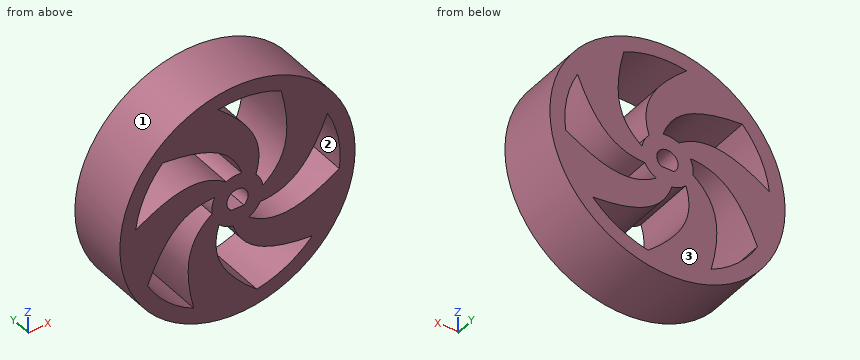
Autodesk Fusion 360 part; units mm, degrees
sketch "Sketch1" plane through (0, 0, 0) normal (0, 1, 0) x (1, 0, 0)
  circle A0 centre (0, 0) radius 2.5
  circle A1 centre (0, 0) radius 27.5
  circle A2 centre (0, 0) radius 6
  circle A3 centre (0, 0) radius 24
  line L0 (0, 0) -> (0, 2.5)
  line L1 (-1.5, 2) -> (1.5, 2)
  line L2 (1.5, 2) -> (1.5, -2)
  line L3 (1.5, -2) -> (-1.5, -2)
  line L4 (-1.5, -2) -> (-1.5, 2)
  line L5 (0, 0) -> (0, -2.5)
  spline S0 degree 5 poles (-10.2165, 21.7169) (-10.3629, 21.1355) (-10.6365, 19.9863) (-10.9889, 18.3035) (-11.3409, 16.1432) (-11.5701, 13.5918) (-11.567, 11.2048) (-11.3076, 8.9989) (-10.7716, 6.9887) (-9.9564, 5.1759) (-8.8773, 3.5497) (-7.8173, 2.3879) (-6.9183, 1.5901) (-6.2735, 1.0903) (-5.9397, 0.8485) knots 0 0 0 0 0 0 0.1 0.2 0.3 0.4 0.5 0.6 0.7 0.8 0.9 1 1 1 1 1 1
  spline S1 degree 5 poles (-21.0302, 11.5643) (-20.8069, 11.0078) (-20.3528, 9.9173) (-19.6488, 8.3487) (-18.6637, 6.3941) (-17.3495, 4.1953) (-15.9439, 2.2659) (-14.4375, 0.6338) (-12.8223, -0.6775) (-11.0972, -1.6649) (-9.2683, -2.3461) (-7.7279, -2.6631) (-6.5316, -2.7801) (-5.7162, -2.8054) (-5.3041, -2.8048) knots 0 0 0 0 0 0 0.1 0.2 0.3 0.4 0.5 0.6 0.7 0.8 0.9 1 1 1 1 1 1
  spline S2 degree 5 poles (-23.8111, -3.0055) (-23.3034, -3.3245) (-22.295, -3.9398) (-20.8034, -4.795) (-18.8576, -5.7973) (-16.502, -6.8037) (-14.2308, -7.5384) (-12.0527, -7.9734) (-9.9752, -8.0848) (-7.9993, -7.8697) (-6.1192, -7.3459) (-4.6867, -6.6968) (-3.6501, -6.0883) (-2.9756, -5.6295) (-2.6425, -5.3868) knots 0 0 0 0 0 0 0.1 0.2 0.3 0.4 0.5 0.6 0.7 0.8 0.9 1 1 1 1 1 1
  spline S3 degree 5 poles (-17.4969, -16.4273) (-16.8987, -16.3869) (-15.7212, -16.292) (-14.0119, -16.1072) (-11.8486, -15.7743) (-9.3513, -15.2039) (-7.082, -14.4633) (-5.0642, -13.535) (-3.318, -12.4041) (-1.8458, -11.0686) (-0.6328, -9.5397) (0.1447, -8.1726) (0.6256, -7.0711) (0.9016, -6.3034) (1.0285, -5.9112) knots 0 0 0 0 0 0 0.1 0.2 0.3 0.4 0.5 0.6 0.7 0.8 0.9 1 1 1 1 1 1
  spline S4 degree 5 poles (-4.4996, -23.5744) (-4.0393, -23.1901) (-3.1425, -22.4212) (-1.8683, -21.267) (-0.3138, -19.7261) (1.3713, -17.7968) (2.7719, -15.8637) (3.8587, -13.9267) (4.6066, -11.9854) (5.0126, -10.0396) (5.0954, -8.0897) (4.9208, -6.5267) (4.6624, -5.3529) (4.4345, -4.5696) (4.3066, -4.1777) knots 0 0 0 0 0 0 0.1 0.2 0.3 0.4 0.5 0.6 0.7 0.8 0.9 1 1 1 1 1 1
  spline S5 degree 5 poles (10.2165, -21.7169) (10.3629, -21.1355) (10.6365, -19.9863) (10.9889, -18.3035) (11.3409, -16.1432) (11.5701, -13.5918) (11.567, -11.2048) (11.3076, -8.9989) (10.7716, -6.9887) (9.9564, -5.1759) (8.8773, -3.5497) (7.8173, -2.3879) (6.9183, -1.5901) (6.2735, -1.0903) (5.9397, -0.8485) knots 0 0 0 0 0 0 0.1 0.2 0.3 0.4 0.5 0.6 0.7 0.8 0.9 1 1 1 1 1 1
  spline S6 degree 5 poles (21.0302, -11.5643) (20.8069, -11.0078) (20.3528, -9.9173) (19.6488, -8.3487) (18.6637, -6.3941) (17.3495, -4.1953) (15.9439, -2.2659) (14.4375, -0.6338) (12.8223, 0.6775) (11.0972, 1.6649) (9.2683, 2.3461) (7.7279, 2.6631) (6.5316, 2.7801) (5.7162, 2.8054) (5.3041, 2.8048) knots 0 0 0 0 0 0 0.1 0.2 0.3 0.4 0.5 0.6 0.7 0.8 0.9 1 1 1 1 1 1
  spline S7 degree 5 poles (23.8111, 3.0055) (23.3034, 3.3245) (22.295, 3.9398) (20.8034, 4.795) (18.8576, 5.7973) (16.502, 6.8037) (14.2308, 7.5384) (12.0527, 7.9734) (9.9752, 8.0848) (7.9993, 7.8697) (6.1192, 7.3459) (4.6867, 6.6968) (3.6501, 6.0883) (2.9756, 5.6295) (2.6425, 5.3868) knots 0 0 0 0 0 0 0.1 0.2 0.3 0.4 0.5 0.6 0.7 0.8 0.9 1 1 1 1 1 1
  spline S8 degree 5 poles (17.4969, 16.4273) (16.8987, 16.3869) (15.7212, 16.292) (14.0119, 16.1072) (11.8486, 15.7743) (9.3513, 15.2039) (7.082, 14.4633) (5.0642, 13.535) (3.318, 12.4041) (1.8458, 11.0686) (0.6328, 9.5397) (-0.1447, 8.1726) (-0.6256, 7.0711) (-0.9016, 6.3034) (-1.0285, 5.9112) knots 0 0 0 0 0 0 0.1 0.2 0.3 0.4 0.5 0.6 0.7 0.8 0.9 1 1 1 1 1 1
  spline S9 degree 5 poles (4.4996, 23.5744) (4.0393, 23.1901) (3.1425, 22.4212) (1.8683, 21.267) (0.3138, 19.7261) (-1.3713, 17.7968) (-2.7719, 15.8637) (-3.8587, 13.9267) (-4.6066, 11.9854) (-5.0126, 10.0396) (-5.0954, 8.0897) (-4.9208, 6.5267) (-4.6624, 5.3529) (-4.4345, 4.5696) (-4.3066, 4.1777) knots 0 0 0 0 0 0 0.1 0.2 0.3 0.4 0.5 0.6 0.7 0.8 0.9 1 1 1 1 1 1
  dimension "d1" = 5
  dimension "d2" = 55
  dimension "d3" = 12
  dimension "d4" = 48
  dimension "d5" = 0.5
  dimension "d6" = 0.5
  dimension "d8" = 360
extrude "Extrude1" add sketch "Sketch1" along normal blind 15 contours A0 L0 L1 | A0 L0 L1 | A1 | A2 | A2 A3 S5 S6 | A2 A3 S7 S8 | A2 A3 S3 S4 | A2 A3 S0 S9 | A2 A3 S1 S2
Work out the finished part from the listing and answer in its coordinate system (mm). Face numbers are marked on the shaded views. Give positions to 0.01 mm unless a question says otherwise; leave off trailing zeros. Write item = value, one per line. Start each with the question number.
(1) Find section A-A on z = 0. Give the number of separate pieces and of enclosed holes in the cut face, and give its area (3 significant figures).
(2) The mould has two halves that part along X. Classify the marked faces 1, 2 and 3: +X half, -X half, draft (parallel to the pull), parting line (faces both ways), or undercut.
(3) Find the intervals of material crossed by probe 1 along X at (y, z) = (9.5, -8.5); probe 2 along Z at (x, y) = (14, 11.5); probe 3 along X at (y, z) = (12.25, 0), in increasing order. Write a range as from..to.
(4) Given pin 1 Ø1.5 at (y, z) = (10, -17.5) entering from +X; pin 2 Ø3.5 at (x, y) = (-0.5, 6) entering from +Z; pin 3 Ø4 at (y, z) = (2, -5.5) entering from +X; pin 4 Ø4 at (x, z) = (-15.5, -9) entering from -Y, each flat-ended and moving along its own axis, determine where each tip first touches the part or whether it passes through.
From the geometry:
q1.separate_pieces = 4
q1.enclosed_holes = 0
q1.area = 480 mm^2
q2.face_1 = parting line
q2.face_2 = undercut
q2.face_3 = draft
q3.probe_1 = -26.15..-19.69, -11.12..-5.03, 0.08..26.15
q3.probe_2 = -23.67..-19.49, -16.08..-7.53, 0.34..23.67
q3.probe_3 = -27.5..-13.59, -6..-2.5, 2.5..13.59, 24..27.5
q4.pin_1 = 21.81
q4.pin_2 = 27.5
q4.pin_3 = 27.28
q4.pin_4 = through
